Here's how the part is built. I have some questions about the finished solid (model axes, mm). Round coordinates to 2 decimals unless told otherwise and drop trailing zeros. Write each loop counter-clockwise with the first axis right and the second up, starting at its lowest first coordinate (ties: lowest second). Pieces come first, ordered by that corner, then holes. Notation, with made-up numbers: (-23.75, 3.25) - (-12.75, 3.25) arc R32 ccw to (-12.75, 39.25) - close; hole circle Ø3 at (18.5, 28). An arc over 180 degrees is marked (long way). Write item = value, one per line. Start each with the question number.
Item 1: If we section it at B-B (x = 0): Please give me the cut outline in (y, z), and give its area (3 significant figures).
Item 2: If we section it at A-A (z = -1.3): Please give me the cut outline in (x, y).
Item 3: For P1, Ø1, axis at y = -10, z = 1.5, coming from the +X side, with a flat end and sliding along its axis, tell me the tip position at first contact or that it passes through.
Item 4: Thinking about a two-plate mould opening in X: for faces 1 (the face through (-0.75, 0.08, -0.04)), 2 (the face through (2.81, -8.185, 2.215)), 3 (the face through (-2.79, -8.32, 2.21)), which applies, pulls with the +X half, pulls with the -X half, needs draft (parallel to the pull), parting line crosses it, or undercut?
Item 5: If I drill on line 1 along Y through (x, z) = (-0.25, -1.5); line 2 along Y through (x, z) = (1, 0.75); line 3 along X through (y, z) = (-1, 1.6), over which ranges is the centre line in solid material (lowest first)? Write a range as [from, to].
```python
from build123d import *

# Parameters (mm, degrees)
F0_R     = 1.75
F1_DEPTH = 2.5
F2_R     = 2
F3_R     = 5
F4_R     = 1


with BuildPart() as f1:
    # F0 (on Top) → F1 (new body, symmetric)
    with BuildSketch(Plane.XY):
        with BuildLine():
            Line((1.8980583428, -14.5959100367), (4.1378631671, -2.8067932611))
            ThreePointArc((4.1378631671, -2.8067932611), (0, 5), (-4.1378631671, -2.8067932611))
            Line((-4.1378631671, -2.8067932611), (-1.8980583428, -14.5959100367))
            Line((-1.8980583428, -14.5959100367), (1.8980583428, -14.5959100367))
        make_face()
        with Locations((1, 0)):
            Circle(F0_R, mode=Mode.SUBTRACT)
    extrude(amount=F1_DEPTH, both=True)

    # F2
    f2_edges = [f1.edges().sort_by_distance(p)[0] for p in [
        (1.898058, -14.59591, 0),
        (-1.898058, -14.59591, 0),
    ]]
    fillet(f2_edges, radius=F2_R)

    # F3
    f3_edges = [f1.edges().sort_by_distance(p)[0] for p in [
        (4.137863, -2.806793, 0),
        (-4.137863, -2.806793, 0),
    ]]
    fillet(f3_edges, radius=F3_R)

    # F4
    f4_edges = [f1.edges().sort_by_distance(p)[0] for p in [
        (0, 5, 2.5),
        (0, 5, -2.5),
    ]]
    fillet(f4_edges, radius=F4_R)


solid = f1.part
```
Reply:
q1.outline = (-14.6, -1.5) arc R1 ccw to (-13.6, -2.5) - (-1.44, -2.5) - (-1.44, 2.5) - (-13.6, 2.5) arc R1 ccw to (-14.6, 1.5) - close; (1.44, -2.5) - (4, -2.5) arc R1 ccw to (5, -1.5) - (5, 1.5) arc R1 ccw to (4, 2.5) - (1.44, 2.5) - close
q1.area = 82.8 mm2
q2.outline = (-4.45, -2.29) arc R5 cw to (-3.98, -3.64) - (-2.21, -12.97) arc R2 ccw to (-0.24, -14.6) - (0.24, -14.6) arc R2 ccw to (2.21, -12.97) - (3.98, -3.64) arc R5 cw to (4.45, -2.29) arc R5 ccw (long way) to start; hole circle Ø3.5 at (1, 0)
q3.P1 = 2.87
q4.face_1 = undercut
q4.face_2 = pulls with the +X half
q4.face_3 = pulls with the -X half
q5.line_1 = [-14.6, -1.22], [1.22, 4.99]
q5.line_2 = [-14.45, -1.75], [1.75, 4.9]
q5.line_3 = [-4.89, -0.44], [2.44, 4.89]
